Here's how the part is built. I have some questions about the finished solid (model axes, mm). Face numbers are marked on the shaded views. Round coordinates to 2 decimals unless told otherwise and drop trailing zeros. Loops run counter-clockwise (first coordinate to the right, second up) from the corner with the lowest first, then second, coordinate; pieces in that order, holes last. Notation, with made-up numbers: M -10.75,55.25 L 4.25,55.25 A7 cw 4.25,64.25 Z; hole C 76.5,17.5 d4. An arc over 180 degrees is marked long. Answer as a JSON object with one key per item and string values.
from build123d import *

# Parameters (mm, degrees)
BOSS_EXTRUDE1_DEPTH = 215.9
SHELL1_T            = -3.175
SKETCH2_R           = 5
CUT_EXTRUDE1_DEPTH  = 439.655867395
LPATTERN1_COUNT     = 7
LPATTERN1_PITCH     = 19.05


with BuildPart() as part:
    # Sketch1 → Boss-Extrude1 (new, symmetric)
    with BuildSketch(Plane.XY):
        Polygon((-12.7, -65.28778243), (6.35, -76.2), (12.7, -76.2), (12.7, 76.2), (-12.7, 76.2), align=None)
    extrude(amount=BOSS_EXTRUDE1_DEPTH, both=True)

    # Shell1
    shell1_openings = [part.faces().sort_by_distance(p)[0] for p in [
        (12.7, 0, 0),
    ]]
    offset(amount=SHELL1_T, openings=shell1_openings, kind=Kind.INTERSECTION)

    # Sketch2 → Cut-Extrude1 (cut, through all)
    with BuildSketch(Plane.XY.offset(215.9)):
        with Locations((3.175, -61.681297072)):
            Circle(SKETCH2_R)
        with Locations((-3.175, -52.156297072)):
            Circle(SKETCH2_R)
    cut_extrude1 = extrude(amount=-CUT_EXTRUDE1_DEPTH, mode=Mode.SUBTRACT)

    # LPattern1: Cut-Extrude1 ×7
    with Locations(*[(0, i * LPATTERN1_PITCH, 0) for i in range(1, LPATTERN1_COUNT)]):
        add(cut_extrude1, mode=Mode.SUBTRACT)


solid = part.part
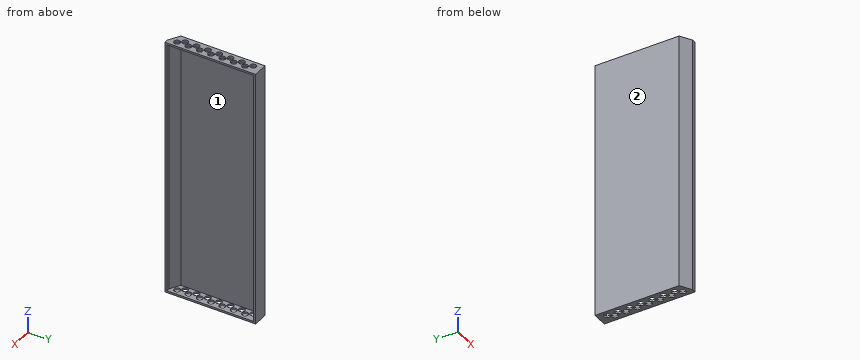
Item 1: I want a section at A-A, the plane z = -164. Please give me the cut outline in (x, y) (3 decimals), then the cut area to 3 significant figures.
Resolved:
{"outline": "M -12.7,-65.288 L 6.35,-76.2 L 12.7,-76.2 L 12.7,-73.025 L 7.195,-73.025 L -9.525,-63.447 L -9.525,73.025 L 12.7,73.025 L 12.7,76.2 L -12.7,76.2 Z", "area": "601 mm²"}
Item 2: If we mould it in two halves opening along Z, with no side actions, what happens to the marked faces 1 and 2? For each: pulls with the +Z half, pulls with the -Z half, needs draft (parallel to the pull), parting line crosses it, or undercut.
Resolved:
{"face 1": "undercut", "face 2": "needs draft"}
Item 3: I'm going to push flat-ended pins straight in: pin 1 Ø8 at (x, y) = (3.18, -61.68) entering from +Z; pin 2 Ø1.5 at (x, z) = (-5, 167) entering from -Y; pin 3 Ø12 at (y, z) = (-19.5, -109) entering from +X (3 decimals); pin 4 Ø6 at (x, z) = (2.5, -110.5) entering from -Y. Where does each tip first touch, or does it pass through?
Resolved:
{"pin 1": "through", "pin 2": "y = -70.13", "pin 3": "x = -9.525", "pin 4": "y = -75.71"}
Item 4: Please list where these lines run through material, in increasing order: probe 1 along Z at (x, y) = (-9, 60) (3 decimals); probe 2 along Y at (x, z) = (11, -87) (3 decimals); probe 3 along X at (y, z) = (-3.5, -32) (3 decimals). Write a range as from..to.
Resolved:
{"probe 1": "-215.9..-212.725, 212.725..215.9", "probe 2": "-76.2..-73.025, 73.025..76.2", "probe 3": "-12.7..-9.525"}
